```python
from build123d import *

# Parameters (mm, degrees)
SKETCH1_W                  = 38.1
SKETCH1_H                  = 8
BOSS_EXTRUDE1_DEPTH        = 5.2
FILLET1_R                  = 4
SKETCH3_R                  = 1.45
CUT_EXTRUDE1_DEPTH         = 5.2
SKETCH4_W                  = 31.85
SKETCH4_H                  = 2.2
CUT_EXTRUDE2_DEPTH         = 5.2
FILLET2_R                  = 1.1
FILLET3_R                  = 1.1
CUT_EXTRUDE3_DEPTH         = 5.2
CUT_EXTRUDE4_START         = -9.612880748
CUT_EXTRUDE4_OUTLINE_W     = 3.2
CUT_EXTRUDE4_OUTLINE_H     = 11
CUT_EXTRUDE4_DEPTH         = 4
SKETCH8_W                  = 3.1
SKETCH8_H                  = 2.2
CUT_EXTRUDE5_DEPTH         = 3.2
SKETCH9_R                  = 2.4
CUT_EXTRUDE6_DEPTH         = 3.2
M2_CLEARANCE_HOLE1_D       = 2.4
F_0_5_0_5_DIAMETER_HOLE1_D = 0.5


# Read off the part's stored shape, not the designer's step: Cut-Extrude4
with BuildPart() as part:
    # Sketch1 → Boss-Extrude1 (new body)
    with BuildSketch(Plane(origin=(0, 0, 0), x_dir=(1, 0, 0), z_dir=(0, 1, 0))):
        with Locations((9.437119252, 0.097413434)):
            Rectangle(SKETCH1_W, SKETCH1_H)
    extrude(amount=BOSS_EXTRUDE1_DEPTH)

    # Fillet1
    fillet1_edges = [part.edges().sort_by_distance(p)[0] for p in [
        (-9.612880748, 2.6, -4.097413434),
        (-9.612880748, 2.6, 3.902586566),
    ]]
    fillet(fillet1_edges, radius=FILLET1_R - 0.0001)  # a hair under: the kernel refuses the full size

    # Sketch3 → Cut-Extrude1 (cut)
    with BuildSketch(Plane(origin=(0, 5.2, 0), x_dir=(1, 0, 0), z_dir=(0, 1, 0))):
        with Locations(Location((-5.612880748, 0.097413434, 0), (0, 0, 270))):
            Circle(SKETCH3_R)
    extrude(amount=-CUT_EXTRUDE1_DEPTH, mode=Mode.SUBTRACT)

    # Sketch4 → Cut-Extrude2 (cut)
    with BuildSketch(Plane(origin=(0, 5.2, 0), x_dir=(1, 0, 0), z_dir=(0, 1, 0))):
        with Locations((12.562119252, -2.802586566)):
            Rectangle(SKETCH4_W, SKETCH4_H)
    extrude(amount=-CUT_EXTRUDE2_DEPTH, mode=Mode.SUBTRACT)

    # Fillet2
    fillet2_edges = [part.edges().sort_by_distance(p)[0] for p in [
        (-3.362880748, 2.6, 1.702586566),
    ]]
    fillet(fillet2_edges, radius=FILLET2_R)

    # Fillet3
    fillet3_edges = [part.edges().sort_by_distance(p)[0] for p in [
        (-3.362880748, 2.6, 3.902586566),
    ]]
    fillet(fillet3_edges, radius=FILLET3_R - 0.0001)  # a hair under: the kernel refuses the full size

    # Sketch5 → Cut-Extrude3 (cut)
    with BuildSketch(Plane(origin=(0, 5.2, 0), x_dir=(1, 0, 0), z_dir=(0, 1, 0))):
        Polygon((28.487119252, 4.097413434), (25.138487691, -1.702586566), (28.487119252, -1.702586566), align=None)
    extrude(amount=-CUT_EXTRUDE3_DEPTH, mode=Mode.SUBTRACT)

    # Cut-Extrude4 outline → Cut-Extrude4 (cut)
    with BuildSketch(Plane.YZ.offset(CUT_EXTRUDE4_START)):
        with Locations((2.6, -0.5)):
            Rectangle(CUT_EXTRUDE4_OUTLINE_W, CUT_EXTRUDE4_OUTLINE_H)
    extrude(amount=CUT_EXTRUDE4_DEPTH, mode=Mode.SUBTRACT)

    # Sketch8 → Cut-Extrude5 (cut)
    with BuildSketch(Plane.XZ.offset(-4.2)):
        with Locations((-4.062880748, 2.802586566)):
            Rectangle(SKETCH8_W, SKETCH8_H)
    extrude(amount=CUT_EXTRUDE5_DEPTH, mode=Mode.SUBTRACT)

    # Sketch9 → Cut-Extrude6 (cut)
    with BuildSketch(Plane.XZ.offset(-4.2)):
        with Locations((-5.612880748, -0.097413434)):
            Circle(SKETCH9_R)
    extrude(amount=CUT_EXTRUDE6_DEPTH, mode=Mode.SUBTRACT)

    # M2 Clearance Hole1 (through all)
    with Locations(Plane(origin=(6.387119252, 2.6, -4.097413434), x_dir=(-1, 0, 0), z_dir=(0, 0, -1))):
        with Locations((0, 0), (-12, 0)):
            Hole(M2_CLEARANCE_HOLE1_D / 2)

    # Ø0.5 (0.5) Diameter Hole1 (through all)
    with Locations(Plane(origin=(24.187119252, 3.539440359, -4.097413434), x_dir=(-1, 0, 0), z_dir=(0, 0, -1))):
        with Locations((0, 0), (0, -2.246762327)):
            Hole(F_0_5_0_5_DIAMETER_HOLE1_D / 2)


solid = part.part
```
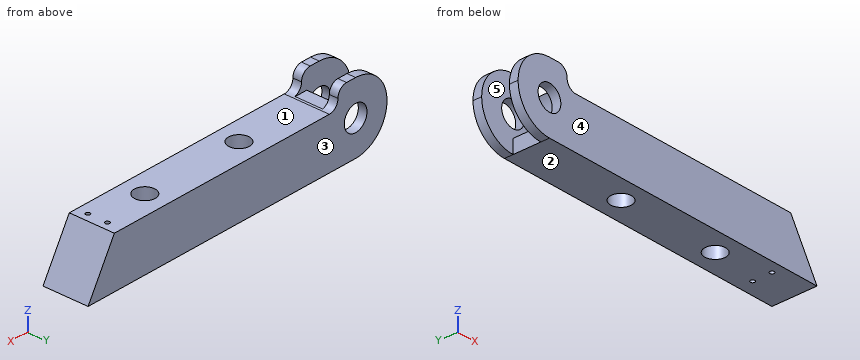
Design review of the part built by this model. Coordinates are the model's own, in mm. Face numbers are marked on the shaded views. A direction names the side the tool comes from. Give positions to 0.01 mm unless a question says otherwise; leave off trailing zeros. Loops run counter-clockwise (first coordinate to the right, second up) from the corner with the lowest first, then second, coordinate; pieces in that order, holes last. Notation, with made-up numbers: (-13, -5.75) -> (6, -5.75) arc R21 cw to (6, 22.25) -> close; hole circle Ø11 at (58, 65). An arc over 180 degrees is marked (long way). Write each question's results on one line, items separated by ' | '.
Q1. Take a section at D-D, the plane z = -2. Write out the cut boundary in (x, y), plus the area to 3 significant figures.
Reply:
outline: (-9.13, 0) -> (27.28, 0) -> (27.28, 5.2) -> (-9.13, 5.2) -> (-9.13, 4.2) -> (-4.15, 4.2) -> (-4.15, 1) -> (-9.13, 1) -> close; hole circle Ø2.4 at (6.39, 2.6); hole circle Ø2.4 at (18.39, 2.6); hole circle Ø0.5 at (24.19, 1.29); hole circle Ø0.5 at (24.19, 3.54) | area: 164 mm²
Q2. Take a section at A-A, the plane y = 2.6. Give the number of separate pieces and of enclosed holes in the cut face, plus the area to 3 significant figures.
Reply:
separate pieces: 3 | enclosed holes: 0 | area: 152 mm²
Q3. The part is to be moulded in two halves that separate along Y. For the marked faces 3, 4 and 5, say which applies: +Y half, -Y half, draft (parallel to the pull), parting line (faces both ways), or undercut.
Reply:
face 3: +Y half | face 4: -Y half | face 5: undercut
Q4. Wall thickness on L1, parallel to Y at x = -3.5, z = 2.5; L2, parallel to X at y = 2.2, z = 0; L3, parallel to X at y = 2.05, z = -2: over which ranges is each line inside the solid? List them lowest first.
Reply:
L1: y = 0 to 1, 4.2 to 5.2 | L2: x = -3.21 to 5.26, 7.52 to 17.26, 19.52 to 26.12 | L3: x = -4.15 to 5.32, 7.45 to 17.32, 19.45 to 27.28
Q5. Take a section at C-C, the plane z = 2.25. Write out the cut boundary in (x, y), plus the area to 3 significant figures.
Reply:
outline: (-8.85, 0) -> (-3.21, 0) -> (-3.21, 1) -> (-8.85, 1) -> close; (-8.85, 4.2) -> (-3.21, 4.2) -> (-3.21, 5.2) -> (-8.85, 5.2) -> close | area: 11.3 mm²
Q6. Machinability: for the marked faces 1 and 2, which of the approach directions +Z, -Z, +X, -X, +Y, -Y give a long, thin tool a straight path to every point of the face, cutting with its end or side? Answer none if there is none.
Reply:
face 1: +Z, +X, +Y, -Y | face 2: -Z, +X, -X, +Y, -Y
Q7. For pin 1 Ø0.8 at (x, y) = (-3, 2) entering from +Z; pin 2 Ø1.3 at (y, z) = (2.5, -3.5) entering from -X; pin 3 Ø1.4 at (x, y) = (6.39, 2.6) entering from +Z, all flat-tipped, find the tip position at first contact; note any pin that passes through.
Reply:
pin 1: stops at z = 1.7 | pin 2: stops at x = -5.61 | pin 3: passes through
Q8. Take a section at B-B, the plane x = 7. Write out the cut boundary in (y, z).
Reply:
outline: (0, -4.1) -> (1.57, -4.1) -> (1.57, 1.7) -> (0, 1.7) -> close; (3.63, -4.1) -> (5.2, -4.1) -> (5.2, 1.7) -> (3.63, 1.7) -> close
